Input: part model. Units: mm. Frame: model coordinates. Coordinates: 2 decimals unless noted, no trailing zeros. Order: outer loops, then holes, each group sorted by start corner. A loop starts at its lowest first (then second) coordinate and runs counter-clockwise, first axis right, second up. Notation, with made-up numbers: (-0.75, -1.5) -> (44.25, -1.5) arc R22 ccw to (44.25, 9.5) -> close; hole circle Ø3 at (16.25, 4). An arc over 180 degrees is marked (long way). Use one line per item in the form item = value. Start each with the question number.
1) Ray query, line 1 along Y through (x, z) = (-16, -516) (3 decimals); line 2 along Z through (x, y) = (-1.75, -0.5); line 3 along Z through (x, y) = (-2.5, 1.5). Return the intervals inside material, ascending.
2) Section query A-A on z = -447. Output: boundary loops of the cut face in (x, y) (3 decimals), then the cut area to 3 significant figures.
3) Pin query (flat end, axial travel): pin 1 (2 mm diameter, centred on x = -1.5, z = -410.5, fed in from -Y) (3 decimals); pin 2 (5.5 mm diameter, centred on x = -8, y = 0.5, fed in from -Z); pin 3 (4 mm diameter, centred on x = 0.5, z = -283.5, fed in from +Y) (3 decimals); pin 4 (1.6 mm diameter, centred on y = 0.5, z = -560.5, fed in from -X). Return the tip coordinate at first contact, or that it passes through.
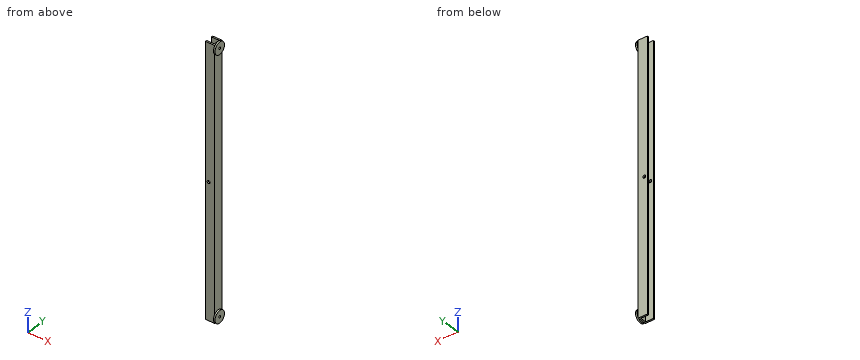
from build123d import *

# Parameters (mm, degrees)
BOSS_EXTRUDE1_DEPTH = 558.8
SKETCH2_R           = 3
CUT_EXTRUDE1_DEPTH  = 558.8
SKETCH4_R           = 2.38125
CUT_EXTRUDE8_DEPTH  = 6.8
BOSS_EXTRUDE3_START = 3.175
SKETCH5_R           = 12.7
SKETCH5_R_2         = 2.38125
BOSS_EXTRUDE3_DEPTH = 3.175


with BuildPart() as part:
    # Sketch1 → Boss-Extrude1 (new body)
    with BuildSketch(Plane.XY):
        Polygon((0, -9.525), (0, 9.525), (-19.01, 9.525), (-19.01, 6.35), (-3.175, 6.35), (-3.175, -6.35), (-19.01, -6.35), (-19.01, -9.525), align=None)
    extrude(amount=-BOSS_EXTRUDE1_DEPTH)

    # Sketch2 → Cut-Extrude1 (cut)
    with BuildSketch(Plane(origin=(0, 9.525, 0), x_dir=(1, 0, 0), z_dir=(0, 1, 0))):
        with Locations(Location((-12.66, 280.013576808, 0), (0, 0, 270))):
            Circle(SKETCH2_R)
    extrude(amount=-CUT_EXTRUDE1_DEPTH, mode=Mode.SUBTRACT)

    # Sketch4 → Cut-Extrude8 (cut)
    with BuildSketch(Plane(origin=(0, 0, 0), x_dir=(0, 0, -1), z_dir=(1, 0, 0))):
        with Locations((9.525, 0)):
            Circle(SKETCH4_R)
        with Locations(Location((549.275, 0, 0), (0, 0, 180))):
            Circle(SKETCH4_R)
    extrude(amount=-CUT_EXTRUDE8_DEPTH, mode=Mode.SUBTRACT)

    # Sketch5 → Boss-Extrude3 (add)
    # profile 1 of 2: a face of its own
    with BuildSketch(Plane(origin=(0, 0, 0), x_dir=(0, 0, -1), z_dir=(1, 0, 0)).offset(BOSS_EXTRUDE3_START)):
        with Locations(Location((9.525, 0, 0), (0, 0, 138.590377891))):
            Circle(SKETCH5_R)
        with Locations((9.525, 0)):
            Circle(SKETCH5_R_2, mode=Mode.SUBTRACT)
    # profile 2 of 2: a face of its own
    with BuildSketch(Plane(origin=(0, 0, 0), x_dir=(0, 0, -1), z_dir=(1, 0, 0)).offset(BOSS_EXTRUDE3_START)):
        with Locations(Location((549.275, 0, 0), (0, 0, 228.590377891))):
            Circle(SKETCH5_R)
        with Locations((549.275, 0)):
            Circle(SKETCH5_R_2, mode=Mode.SUBTRACT)
    extrude(amount=-BOSS_EXTRUDE3_DEPTH)


solid = part.part
Answers below:
q1.line_1 = -9.525 to -6.35, 6.35 to 9.525
q1.line_2 = -558.8 to -551.6, -546.95 to -11.85, -7.2 to 0
q1.line_3 = -558.8 to -551.12, -547.43 to -11.37, -7.68 to 0
q2.outline = (-19.01, -9.525) -> (0, -9.525) -> (0, 9.525) -> (-19.01, 9.525) -> (-19.01, 6.35) -> (-3.175, 6.35) -> (-3.175, -6.35) -> (-19.01, -6.35) -> close
q2.area = 161 mm^2
q3.pin_1 = -9.525
q3.pin_2 = through
q3.pin_3 = 9.525
q3.pin_4 = 0
